The listing builds one solid part. Answer for the finished solid, in the listing's coordinates (mm). A direction names the side the tool comes from. Coordinates: 2 decimals unless noted, no trailing zeros. Order: outer loops, then holes, each group sorted by start corner. A loop starts at its lowest first (then second) coordinate and runs counter-clockwise, first axis right, second up. Notation, with made-up numbers: (11, 75.25) -> (26, 75.25) arc R27 cw to (26, 100.25) -> close; hole circle Ø2 at (3.25, 51). An arc over 180 degrees is marked (long way). Put each result on its own line as item: value. Start each with the question number.
```python
from build123d import *

# Parameters (mm, degrees)
SKETCH_1_W          = 20
SKETCH_1_H          = 20
SKETCH_1_W_2        = 18
SKETCH_1_H_2        = 18
EXTRUDE_1_DEPTH     = 900
SKETCH_2_R          = 2.75
CUT_EXTRUDE_1_DEPTH = 37
SKETCH_3_R          = 2.1
CUT_EXTRUDE_2_DEPTH = 37
SKETCH_4_R          = 2.1
CUT_EXTRUDE_3_DEPTH = 37


with BuildPart() as part:
    # 草图1 → 拉伸-薄壁1 (new body)
    with BuildSketch(Plane.XY):
        with Locations((10, -10)):
            Rectangle(SKETCH_1_W, SKETCH_1_H)
        with Locations((10, -10)):
            Rectangle(SKETCH_1_W_2, SKETCH_1_H_2, mode=Mode.SUBTRACT)
    extrude(amount=EXTRUDE_1_DEPTH)

    # 草图2 → 切除-拉伸1 (cut)
    with BuildSketch(Plane(origin=(0, 0, 0), x_dir=(1, 0, 0), z_dir=(0, 1, 0))):
        with Locations(Location((11, -35, 0), (0, 0, 270))):
            Circle(SKETCH_2_R)
        with Locations(Location((11, -55, 0), (0, 0, 270))):
            Circle(SKETCH_2_R)
        with Locations(Location((11, -845, 0), (0, 0, 90))):
            Circle(SKETCH_2_R)
        with Locations(Location((11, -865, 0), (0, 0, 90))):
            Circle(SKETCH_2_R)
    extrude(amount=-CUT_EXTRUDE_1_DEPTH, mode=Mode.SUBTRACT)

    # 草图3 → 切除-拉伸2 (cut)
    with BuildSketch(Plane(origin=(0, 0, 0), x_dir=(1, 0, 0), z_dir=(0, 1, 0))):
        with Locations(Location((10, -175, 0), (0, 0, 270))):
            Circle(SKETCH_3_R)
        with Locations(Location((10, -220, 0), (0, 0, 270))):
            Circle(SKETCH_3_R)
        with Locations(Location((10, -265, 0), (0, 0, 270))):
            Circle(SKETCH_3_R)
    extrude(amount=-CUT_EXTRUDE_2_DEPTH, mode=Mode.SUBTRACT)

    # 草图4 → 切除-拉伸3 (cut)
    with BuildSketch(Plane(origin=(0, 0, 0), x_dir=(1, 0, 0), z_dir=(0, 1, 0))):
        with Locations(Location((10, -780, 0), (0, 0, 270))):
            Circle(SKETCH_4_R)
        with Locations(Location((10, -730, 0), (0, 0, 270))):
            Circle(SKETCH_4_R)
        with Locations(Location((10, -680, 0), (0, 0, 270))):
            Circle(SKETCH_4_R)
        with Locations(Location((10, -630, 0), (0, 0, 270))):
            Circle(SKETCH_4_R)
        with Locations(Location((10, -580, 0), (0, 0, 270))):
            Circle(SKETCH_4_R)
    extrude(amount=-CUT_EXTRUDE_3_DEPTH, mode=Mode.SUBTRACT)


solid = part.part
```
(1) For a pull along Y with two mould halves and no side action, classify faces 3 (the flat face through (1, -10, 444)), 4 (the flat face through (10, -20, 444)), 5 (the flat face through (9.2, -19.6, 900)) as released by +Y, released by -Y, zero draft, split by the parting line, or undercut.
(2) A tool of negligible diameter and unlimited length cuts with its end or side. For faces 1 (the flat face through (20, -10, 444)), 2 (the flat face through (19, -10, 444)), from which of +Z, -Z, +X, -X, +Y, -Y can it reach the whole face along a straight path? Write none if from no direction.
(3) Find the intervals of material crossed by L1, parallel to Y at x = 11.5, z = 86.5; L2, parallel to X at y = -5.5, z = 739; L3, parallel to X at y = -0.8, z = 175, in increasing order.
(4) The part is cut by section A-A on y = -13.75. Determine the outline of the cut face in (x, z), plus the area to 3 significant figures.
(5) The part is cut by section B-B on z = 328. Determine the outline of the cut face in (x, y).
Worked out:
1. face 3: undercut
1. face 4: released by -Y
1. face 5: zero draft
2. face 1: +Z, -Z, +X, +Y, -Y
2. face 2: +Z, -Z
3. L1: -20 to -19, -1 to 0
3. L2: 0 to 1, 19 to 20
3. L3: 0 to 7.9, 12.1 to 20
4. outline: (0, 0) -> (1, 0) -> (1, 900) -> (0, 900) -> close; (19, 0) -> (20, 0) -> (20, 900) -> (19, 900) -> close
4. area: 1,800 mm2
5. outline: (0, -20) -> (20, -20) -> (20, 0) -> (0, 0) -> close; hole (1, -19) -> (19, -19) -> (19, -1) -> (1, -1) -> close
